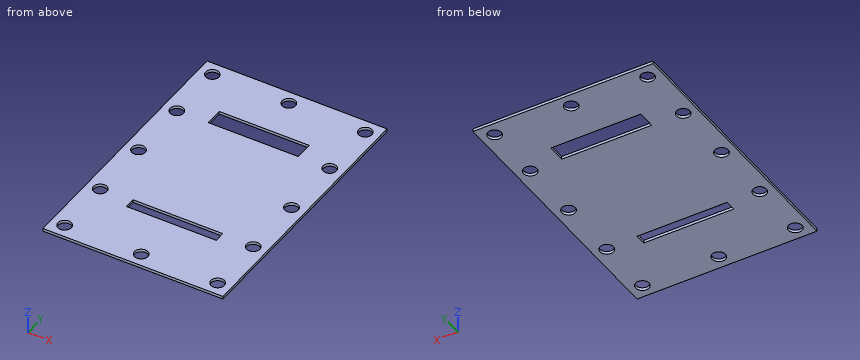
from build123d import *

# Parameters (mm, degrees)
F0_W     = 100
F0_H     = 150
F1_DEPTH = 1.5875
F2_R     = 3.75
F3_DEPTH = 25
F4_W     = 50
F4_H     = 6
F5_DEPTH = 25
F6_W     = 50
F6_H     = 10
F7_DEPTH = 25


# Not quite as in the source:
# - a feature names something its author has since deleted; it is built from what else it names


with BuildPart() as f1:
    # F0 (on Top) → F1 (new body)
    with BuildSketch(Plane.XY):
        Rectangle(F0_W, F0_H)
    extrude(amount=F1_DEPTH)

    # F2 (on face) → F3 (cut)
    with BuildSketch(Plane.XY.offset(1.5875)):
        with Locations((-42.5, 67.5)):
            Circle(F2_R)
        with Locations((-42.5, 0)):
            Circle(F2_R)
        with Locations((-42.5, -35)):
            Circle(F2_R)
        with Locations((-42.5, -67.5)):
            Circle(F2_R)
        with Locations((0, -67.5)):
            Circle(F2_R)
        with Locations((-42.5, 35)):
            Circle(F2_R)
        with Locations((42.5, -67.5)):
            Circle(F2_R)
        with Locations((42.5, -35)):
            Circle(F2_R)
        with Locations((42.5, 0)):
            Circle(F2_R)
        with Locations((42.5, 35)):
            Circle(F2_R)
        with Locations((42.5, 67.5)):
            Circle(F2_R)
        with Locations((0, 67.5)):
            Circle(F2_R)
    extrude(amount=-F3_DEPTH, mode=Mode.SUBTRACT)

    # F4 (on face) → F5 (cut)
    with BuildSketch(Plane.XY.offset(1.5875)):
        with Locations((0, -37)):
            Rectangle(F4_W, F4_H)
    extrude(amount=-F5_DEPTH, mode=Mode.SUBTRACT)

    # F6 (on face) → F7 (cut)
    with BuildSketch(Plane.XY.offset(1.5875)):
        with Locations((0, 40)):
            Rectangle(F6_W, F6_H)
    extrude(amount=-F7_DEPTH, mode=Mode.SUBTRACT)


solid = f1.part
Could you check a few things on this model? Use its own coordinates, in mm. Give positions to 0.01 mm unless a question says otherwise; leave off trailing zeros. Order: outer loops, then holes, each group sorted by start corner. A loop starts at its lowest first (then second) coordinate and runs counter-clockwise, first axis right, second up. Notation, with made-up numbers: M -34,40.5 L -27,40.5 A23 cw -27,58.5 Z; hole C 84,35 d5. An arc over 180 degrees is marked long. One line per question, with ' | ' between items.
1. I want a section at C-C (y = 0). List the corners of the cut face in (x, z) for me, and give its area (3 significant figures).
Results:
outline: M -50,0 L -46.25,0 L -46.25,1.59 L -50,1.59 Z; M -38.75,0 L 38.75,0 L 38.75,1.59 L -38.75,1.59 Z; M 46.25,0 L 50,0 L 50,1.59 L 46.25,1.59 Z | area: 135 mm²
2. I want a section at A-A (x = -20). List the corners of the cut face in (y, z) for me, and give its area (3 significant figures).
Results:
outline: M -75,0 L -40,0 L -40,1.59 L -75,1.59 Z; M -34,0 L 35,0 L 35,1.59 L -34,1.59 Z; M 45,0 L 75,0 L 75,1.59 L 45,1.59 Z | area: 213 mm²
3. I'm going to push a flat-ended pin straight in: pin 1 (7 mm diameter, centred on x = 42.5, y = 35, fed in from -Z). Where does the tip first touch, or does it pass through?
Results:
pin 1: through
4. I want a section at D-D (z = 0.25). Give the number of separate pieces and of enclosed holes in the cut face, and give its area (3 significant figures).
Results:
separate pieces: 1 | enclosed holes: 14 | area: 13,700 mm²
5. I want a section at B-B (x = 42.5). List the corners of the cut face in (y, z) for me.
Results:
outline: M -75,0 L -71.25,0 L -71.25,1.59 L -75,1.59 Z; M -63.75,0 L -38.75,0 L -38.75,1.59 L -63.75,1.59 Z; M -31.25,0 L -3.75,0 L -3.75,1.59 L -31.25,1.59 Z; M 3.75,0 L 31.25,0 L 31.25,1.59 L 3.75,1.59 Z; M 38.75,0 L 63.75,0 L 63.75,1.59 L 38.75,1.59 Z; M 71.25,0 L 75,0 L 75,1.59 L 71.25,1.59 Z
6. If I drill on line 1 (Y direction, x = -42.5, z = 0.45); line 2 (Y direction, x = 0, z = 0.7); line 3 (X direction, y = -35.5, z = 0.85), over which ranges is the centre line in solid material (lowest first)?
Results:
line 1: -75 to -71.25, -63.75 to -38.75, -31.25 to -3.75, 3.75 to 31.25, 38.75 to 63.75, 71.25 to 75 | line 2: -75 to -71.25, -63.75 to -40, -34 to 35, 45 to 63.75, 71.25 to 75 | line 3: -50 to -46.22, -38.78 to -25, 25 to 38.78, 46.22 to 50
